```python
from build123d import *

# Parameters (mm, degrees)
F1_DEPTH  = 17.78
F2_W      = 6.35
F2_H      = 6.1400055
F3_DEPTH  = 9.525
F2_W_2    = 30.48
F4_DEPTH  = 4.7625
F5_R      = 5.5687296145
F6_DEPTH  = 4.7625
F7_DEPTH  = 17.4625
F8_DEPTH  = 25.4
F9_DEPTH  = 15.875
F10_W     = 9.525
F10_H     = 5.08
F10_H_2   = 3.175
F11_DEPTH = 43.18


# Not quite as in the source:
# - a length typed as a fraction of an inch, garbled in the dataset ("3 / 203.2 mm" for 3/8 in), is restored
# - a feature names something its author has since deleted; it is built from what else it names


with BuildPart() as f1:
    # F0 (on Top) → F1 (new body)
    with BuildSketch(Plane.XY):
        Polygon((-39.878, 21.59), (-39.878, 0), (-39.878, -21.59), (39.878, -21.59), (39.878, 0), (39.878, 21.59), align=None)
    extrude(amount=F1_DEPTH)

    # F2 (on face) → F3 (cut)
    with BuildSketch(Plane(origin=(-39.878, 0, 0), x_dir=(0, -1, 0), z_dir=(-1, 0, 0))):
        with Locations((-18.415, 3.07000275)):
            Rectangle(F2_W, F2_H)
        with Locations((18.415, 3.07000275)):
            Rectangle(F2_W, F2_H)
        with BuildLine():
            Line((-21.59, 17.78), (-21.59, 12.28))
            Line((-21.59, 12.28), (-19.9, 12.28))
            ThreePointArc((-19.9, 12.28), (-18.2890872965, 16.1690872965), (-14.4, 17.78))
            Line((-14.4, 17.78), (-21.59, 17.78))
        make_face()
        with BuildLine():
            Line((-2.13, 17.78), (-14.4, 17.78))
            ThreePointArc((-14.4, 17.78), (-10.5109127035, 16.1690872965), (-8.9, 12.28))
            Line((-8.9, 12.28), (-7.63, 12.28))
            ThreePointArc((-7.63, 12.28), (-6.0190872965, 16.1690872965), (-2.13, 17.78))
        make_face()
        with BuildLine():
            Line((15.64, 12.28), (21.59, 12.28))
            Line((21.59, 12.28), (21.59, 17.78))
            Line((21.59, 17.78), (10.14, 17.78))
            ThreePointArc((10.14, 17.78), (14.0290872965, 16.1690872965), (15.64, 12.28))
        make_face()
        with BuildLine():
            Line((10.14, 17.78), (-2.13, 17.78))
            ThreePointArc((-2.13, 17.78), (1.7590872965, 16.1690872965), (3.37, 12.28))
            Line((3.37, 12.28), (4.64, 12.28))
            ThreePointArc((4.64, 12.28), (6.2509127035, 16.1690872965), (10.14, 17.78))
        make_face()
    extrude(amount=-F3_DEPTH, mode=Mode.SUBTRACT)

    # F2 (on face) → F4 (cut)
    with BuildSketch(Plane(origin=(-39.878, 0, 0), x_dir=(0, -1, 0), z_dir=(-1, 0, 0))):
        with Locations((0, 3.07000275)):
            Rectangle(F2_W_2, F2_H)
        with BuildLine():
            Line((-21.59, 12.28), (-21.59, 6.1400055))
            Line((-21.59, 6.1400055), (-15.24, 6.1400055))
            Line((-15.24, 6.1400055), (15.24, 6.1400055))
            Line((15.24, 6.1400055), (21.59, 6.1400055))
            Line((21.59, 6.1400055), (21.59, 12.28))
            Line((21.59, 12.28), (15.64, 12.28))
            ThreePointArc((15.64, 12.28), (10.14, 6.78), (4.64, 12.28))
            Line((4.64, 12.28), (3.37, 12.28))
            ThreePointArc((3.37, 12.28), (-2.13, 6.78), (-7.63, 12.28))
            Line((-7.63, 12.28), (-8.9, 12.28))
            ThreePointArc((-8.9, 12.28), (-14.4, 6.78), (-19.9, 12.28))
            Line((-19.9, 12.28), (-21.59, 12.28))
        make_face()
    extrude(amount=-F4_DEPTH, mode=Mode.SUBTRACT)

    # F5 (on face) → F6 (cut)
    with BuildSketch(Plane.YZ.offset(39.878)):
        with BuildLine():
            Line((14.1410236641, 17.78), (-14.1410236641, 17.78))
            Line((-14.1410236641, 17.78), (-14.1410236641, 13.925705291))
            ThreePointArc((-14.1410236641, 13.925705291), (-8.0583664109, 15.3792022386), (-3.3407865054, 11.2736191532))
            Line((-3.3407865054, 11.2736191532), (3.3407865054, 11.2736191532))
            ThreePointArc((3.3407865054, 11.2736191532), (8.0583664109, 15.3792022386), (14.1410236641, 13.925705291))
            Line((14.1410236641, 13.925705291), (14.1410236641, 17.78))
        make_face()
        with BuildLine():
            ThreePointArc((-14.1410236641, 13.925705291), (-16.3223765845, 10.3766090016), (-16.0373890971, 6.2205090068))
            ThreePointArc((-16.0373890971, 6.2205090068), (-15.0623054432, 4.5248800343), (-13.6467597401, 3.175))
            ThreePointArc((-13.6467597401, 3.175), (-7.7553416056, 2.1900909973), (-3.3407865054, 6.2138400758))
            Line((-3.3407865054, 6.2138400758), (3.3407865054, 6.2138400758))
            ThreePointArc((3.3407865054, 6.2138400758), (7.7553416056, 2.1900909973), (13.6467597401, 3.175))
            ThreePointArc((13.6467597401, 3.175), (15.0623054432, 4.5248800343), (16.0373890971, 6.2205090068))
            ThreePointArc((16.0373890971, 6.2205090068), (16.3223765845, 10.3766090016), (14.1410236641, 13.925705291))
            ThreePointArc((14.1410236641, 13.925705291), (8.0583664109, 15.3792022386), (3.3407865054, 11.2736191532))
            Line((3.3407865054, 11.2736191532), (-3.3407865054, 11.2736191532))
            ThreePointArc((-3.3407865054, 11.2736191532), (-8.0583664109, 15.3792022386), (-14.1410236641, 13.925705291))
        make_face()
        with Locations((-9.6877607201, 8.7437296145)):
            Circle(F5_R, mode=Mode.SUBTRACT)
        with Locations((9.6877607201, 8.7437296145)):
            Circle(F5_R, mode=Mode.SUBTRACT)
    extrude(amount=-F6_DEPTH, mode=Mode.SUBTRACT)

    # F5 (on face) → F7 (cut)
    with BuildSketch(Plane.YZ.offset(39.878)):
        with BuildLine():
            ThreePointArc((-15.24, 3.175), (-16.1699359684, 0.9299359711), (-18.4149999962, 0))
            Line((-18.4149999962, 0), (-12.0420521125, 0))
            Line((-12.0420521125, 0), (18.41500001, 0))
            ThreePointArc((18.41500001, 0), (16.1699359733, 0.9299359662), (15.24, 3.175))
            Line((15.24, 3.175), (13.6467597401, 3.175))
            ThreePointArc((13.6467597401, 3.175), (7.7553416056, 2.1900909973), (3.3407865054, 6.2138400758))
            Line((3.3407865054, 6.2138400758), (-3.3407865054, 6.2138400758))
            ThreePointArc((-3.3407865054, 6.2138400758), (-7.7553416056, 2.1900909973), (-13.6467597401, 3.175))
            Line((-13.6467597401, 3.175), (-15.24, 3.175))
        make_face()
    extrude(amount=-F7_DEPTH, mode=Mode.SUBTRACT)

    # F5 (on face) → F8 (cut)
    with BuildSketch(Plane.YZ.offset(39.878)):
        with BuildLine():
            Line((-21.59, 17.78), (-21.59, 3.175))
            ThreePointArc((-21.59, 3.175), (-20.3164565142, 5.7176537563), (-17.5175035436, 6.2205090068))
            Line((-17.5175035436, 6.2205090068), (-16.0373890971, 6.2205090068))
            ThreePointArc((-16.0373890971, 6.2205090068), (-16.3223765845, 10.3766090016), (-14.1410236641, 13.925705291))
            Line((-14.1410236641, 13.925705291), (-14.1410236641, 17.78))
            Line((-14.1410236641, 17.78), (-21.59, 17.78))
        make_face()
        with BuildLine():
            Line((21.59, 17.78), (14.1410236641, 17.78))
            Line((14.1410236641, 17.78), (14.1410236641, 13.925705291))
            ThreePointArc((14.1410236641, 13.925705291), (16.3223765845, 10.3766090016), (16.0373890971, 6.2205090068))
            Line((16.0373890971, 6.2205090068), (17.5175035436, 6.2205090068))
            ThreePointArc((17.5175035436, 6.2205090068), (20.3164565142, 5.7176537563), (21.59, 3.175))
            Line((21.59, 3.175), (21.59, 17.78))
        make_face()
    extrude(amount=-F8_DEPTH, mode=Mode.SUBTRACT)

    # F5 (on face) → F9 (cut)
    with BuildSketch(Plane.YZ.offset(39.878)):
        with BuildLine():
            Line((-21.59, 3.175), (-21.59, 0))
            Line((-21.59, 0), (-18.4149999962, 0))
            ThreePointArc((-18.4149999962, 0), (-20.6600640289, 0.9299359684), (-21.59, 3.175))
        make_face()
        with BuildLine():
            ThreePointArc((-15.24, 3.175), (-16.1699359684, 0.9299359711), (-18.4149999962, 0))
            Line((-18.4149999962, 0), (-12.0420521125, 0))
            Line((-12.0420521125, 0), (18.41500001, 0))
            ThreePointArc((18.41500001, 0), (16.1699359733, 0.9299359662), (15.24, 3.175))
            Line((15.24, 3.175), (13.6467597401, 3.175))
            ThreePointArc((13.6467597401, 3.175), (7.7553416056, 2.1900909973), (3.3407865054, 6.2138400758))
            Line((3.3407865054, 6.2138400758), (-3.3407865054, 6.2138400758))
            ThreePointArc((-3.3407865054, 6.2138400758), (-7.7553416056, 2.1900909973), (-13.6467597401, 3.175))
            Line((-13.6467597401, 3.175), (-15.24, 3.175))
        make_face()
        with BuildLine():
            ThreePointArc((21.59, 3.175), (20.6600640338, 0.9299359733), (18.41500001, 0))
            Line((18.41500001, 0), (21.59, 0))
            Line((21.59, 0), (21.59, 3.175))
        make_face()
    extrude(amount=-F9_DEPTH, mode=Mode.SUBTRACT)

    # F10 (on face) → F11 (join)
    with BuildSketch(Plane.XZ.offset(21.59)):
        with BuildLine():
            ThreePointArc((24.003, 8.255), (21.2131920908, 14.9901920908), (14.478, 17.78))
            Line((14.478, 17.78), (14.478, 8.255))
            Line((14.478, 8.255), (24.003, 8.255))
        make_face()
        with Locations((19.2405, 5.715)):
            Rectangle(F10_W, F10_H)
        with Locations((19.2405, 1.5875)):
            Rectangle(F10_W, F10_H_2)
    extrude(amount=-F11_DEPTH)


solid = f1.part
```
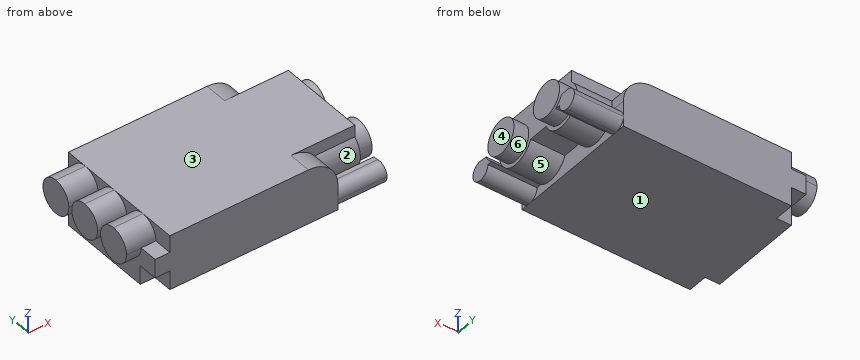
Work out the finished part from the listing and answer in its coordinate system (mm). Face numbers are marked on the shaded views. A direction names the side the tool comes from. Coordinates: 2 decimals unless noted, no trailing zeros. Loops run counter-clockwise (first coordinate to the right, second up) from the corner with the lowest first, then second, coordinate; pieces in that order, holes last. Notation, with made-up numbers: M 71,46 L 113,46 A15 cw 113,55 Z; hole C 0,9.5 d7. An arc over 180 degrees is marked long. Use CSV: the item, a comma, the result in double quotes. Start each with the question number.
(1) Given pin 1 Ø1.8 at (x, y) = (31.5, -15) entering from -Z; pin 2 Ø4.5 at (y, z) = (-17.5, 16.5) entering from -X; pin 3 Ø2.5 at (x, z) = (-33.5, 3.5) entering from -Y, each flat-ended and moving along its own axis, determine where each tip first touches the part or whether it passes through.
(2) Find section C-C, the plane y = -11. Give the vertices of the cut face in (x, z), then the cut area to 3 significant figures.
(3) For a pull along Z with two mould halves and no side action, classify the marked faces 1, 2 and 3 as +Z half, -Z half, draft (parallel to the pull), parting line (faces both ways), or undercut.
(4) Find section B-B, the plane z = 1. Give the vertices of the cut face in (x, y), then the cut area to 3 significant figures.
(5) Consider line 1 (Y direction, x = -30.5, z = 13.5); line 2 (Z direction, x = 32.5, y = -14) (3 decimals); line 3 (Y direction, x = 29, z = 6). Determine where each line is inside the solid, lowest interval first.
(6) For the marked faces 4, 5 and 6, determine the directions among +Z, -Z, +X, -X, +Y, -Y from which every point of the face is accessible in a straight line to the end or side of a thin tool.
Recorded:
1,pin 1,"stops at z = 1.24"
1,pin 2,"stops at x = -30.35"
1,pin 3,"stops at y = -15.24"
2,outline,"M -39.88,6.85 L -35.12,6.85 L -35.12,0 L 24,0 L 24,2.04 L 35.12,2.04 L 35.12,3.33 L 39.88,3.33 L 39.88,14.16 L 35.12,14.16 L 35.12,17.78 L -30.35,17.78 L -30.35,17.71 L -39.88,17.71 Z"
2,area,"1,330 mm^2"
3,face 1,"-Z half"
3,face 2,"undercut"
3,face 3,"+Z half"
4,outline,"M -35.12,-15.24 L -30.35,-15.24 L -30.35,-21.59 L 24,-21.59 L 24,-20.73 L 39.88,-20.73 L 39.88,-16.1 L 24,-16.1 L 24,16.1 L 39.88,16.1 L 39.88,20.73 L 24,20.73 L 24,21.59 L -30.35,21.59 L -30.35,15.24 L -35.12,15.24 Z"
4,area,"2,640 mm^2"
5,line 1,"y = -15.5 to -4.78, -3.23 to 7.49, 9.04 to 19.76"
5,line 2,"z = 3.175 to 17.78"
5,line 3,"y = -19.86 to -3.43, 3.43 to 19.86"
6,face 4,"+Z, -Z, +X, +Y, -Y"
6,face 5,"-Z, +X"
6,face 6,"+X"
